Part model, mm, in its own coordinate system. Give positions to 0.01 mm unless a question says otherwise; leave off trailing zeros. Write each loop counter-clockwise with the first axis right and the second up, starting at its lowest first coordinate (ties: lowest second). Pieces come first, ordered by that corner, then holes. Notation, with made-up numbers: (-34, -18.75) - (25, -18.75) arc R28 ccw to (25, 4.25) - close; hole circle Ø3 at (30.5, 57.5). An arc over 180 degrees is marked (long way). Answer as a JSON object with one key per item and string values. Group by question number.
Autodesk Inventor part; units mm, degrees
ref_plane "YZ Plane" through (0, 0, 0) normal (1, 0, 0) x (0, 1, 0)
ref_plane "XZ Plane" through (0, 0, 0) normal (0, 1, 0) x (-1, 0, 0)
ref_plane "XY Plane" through (0, 0, 0) normal (0, 0, 1) x (1, 0, 0)
sketch "Sketch1" plane through (0, 0, 0) normal (0, 0, 1) x (1, 0, 0)
  line L0 (0, 0) -> (-34.0118, 0)
  line L1 (0, 0) -> (0, 29.864)
  circle A0 centre (-101.344, 0) radius 5.25
  arc A1 (-91.3761, 8.7294) -> (-91.3761, -8.7294) centre (-101.344, 0) ccw
  arc A2 (86.7622, -9.4286) -> (86.7622, 9.4286) centre (100.303, 0) ccw
  line L2 (-85.3577, 6) -> (80.197, 6)
  line L3 (-85.3577, -6) -> (80.197, -6)
  arc A3 (-91.3761, 8.7294) -> (-85.3577, 6) centre (-85.3577, 14) ccw
  arc A4 (-85.3577, -6) -> (-91.3761, -8.7294) centre (-85.3577, -14) ccw
  arc A5 (80.197, 6) -> (86.7622, 9.4286) centre (80.197, 14) ccw
  arc A6 (86.7622, -9.4286) -> (80.197, -6) centre (80.197, -14) ccw
  circle A7 centre (100.303, 0) radius 8.5
  point P0 (-89.5303, 6)
  point P1 (84.9326, 6)
  point P2 (-89.5303, -6)
  point P3 (84.9326, -6)
  dimension "d0" = 201.647
  dimension "d1" = 10.5
  dimension "d2" = 8
  dimension "d4" = 12
  dimension "d5" = 8
  dimension "d9" = 17
  dimension "d10" = 8
extrude "Extrusion1" add sketch "Sketch1" along normal blind 3
fillet "Fillet1" radius 2 1 edges at (91.803, 0, 3)
properties part number "destek bağlantısı" material "Polystyrene"
1) Drill centre lines: line 1 along X through (y, z) = (-0.5, 1); line 2 along Y through (x, z) = (37, 1.7); line 3 along X through (y, z) = (-3.5, 0.3). Where is each one in solid material? Low to high. Write a range as from..to.
2) Saw through at A-A (y = 0). List the corners of the cut face in (x, z).
3) Drop flat-ended pins along their axis: P1, Ø0.9, axis at x = 4, z = 2, coming from the +Y side; P2, Ø1.5, axis at x = -29.5, z = 1, coming from the -Y side. Give the stop position or say it passes through.
4) Saw through at B-B (z = 2.4). List the corners of the cut face in (x, y).
5) Saw through at C-C (x = -58.5). List the corners of the cut face in (y, z).
6) Two-plate mould, pull along X, no slides. Class faces 1 (the flat face through (1, -1, 0)), 2 (the cylindrical face through (116.793, 0.585, 1.479)): +X half, -X half, draft (parallel to the pull), parting line (faces both ways), or undercut.
Checks:
{
 "1": {"line 1": "-114.58..-106.57, -96.12..91.82, 108.79..116.8", "line 2": "-6..6", "line 3": "-114.12..-105.26, -97.43..92.56, 108.05..116.43"},
 "2": {"outline": "(-114.59, 0) - (-106.59, 0) - (-106.59, 3) - (-114.59, 3) - close; (-96.09, 0) - (91.8, 0) - (91.8, 1) arc R2 ccw to (89.8, 3) - (-96.09, 3) - close; (108.8, 0) - (116.8, 0) - (116.8, 3) - (110.8, 3) arc R2 ccw to (108.8, 1) - close"},
 "3": {"P1": "y = 6", "P2": "y = -6"},
 "4": {"outline": "(-91.38, -8.73) arc R8 cw to (-85.36, -6) - (80.2, -6) arc R8 cw to (86.76, -9.43) arc R16.5 ccw (long way) to (86.76, 9.43) arc R8 cw to (80.2, 6) - (-85.36, 6) arc R8 cw to (-91.38, 8.73) arc R13.25 ccw (long way) to start; hole circle Ø10.5 at (-101.34, 0); hole circle Ø18.14 at (100.3, 0)"},
 "5": {"outline": "(-6, 0) - (6, 0) - (6, 3) - (-6, 3) - close"},
 "6": {"face 1": "draft", "face 2": "undercut"}
}
